Job drawing, mm, ordinate dimensions from the low corner. One solid piece. A direction names the side the tool comes from. Round coordinates to 2 decimals unless told otherwise and drop trailing zeros. Write each loop counter-clockwise with the first axis right and the second up, starting at its lowest first coordinate (ties: lowest second). Pieces come first, ordered by that corner, then holes. Notation, with made-up numbers: (24.5, 3.5) -> (41.5, 3.5) arc R19 ccw to (41.5, 27.5) -> close; hole circle Ø11 at (-16.5, -31). An arc over 180 degrees is marked (long way). Use CSV: the item, a comma, the result in double quotes. Start each with the question number.
(1) Saw through at D-D (z = 40). Give the cut face in (x, y), plus the area to 3 significant figures.
(2) Saw through at C-C (y = 14.5). Give the cut face in (x, z).
(3) Saw through at B-B (x = 51). Give the cut face in (y, z).
(4) Probe line 1 (Y direction, x = 5, z = 18); line 2 (Z direction, x = 14, y = 12.5); line 3 (Y direction, x = 63.5, z = 56.15). List the from-to ranges inside material, lowest first. Write a range as [from, to].
(5) Two-plate mould, pull along Z, no slides. Class the marked faces 5, 6 and 7: released by +Z, released by -Z, zero draft, split by the parting line, or undercut.
(6) Which spindle directions (+Z, -Z, +X, -X, +Y, -Y) get a long thin tool onto all of the face, cutting with end or side? Do the marked faces 1, 2, 3 and 4. Say none if no direction does.
(7) Saw through at A-A (x = 5). Give the cut face in (y, z), plus the area to 3 significant figures.
(8) Drop flat-ended pins along their axis: pin 1 (5.5 mm diameter, centred on x = 5, y = 14.5, fed in from +Z); pin 2 (12 mm diameter, centred on x = 23.5, z = 49, fed in from -Y); pin 3 (6 mm diameter, centred on y = 13.5, z = 44, fed in from +X); pin 4 (5.5 mm diameter, centred on y = 4.5, z = 31.5, fed in from -X). Give the stop position or say it passes through.
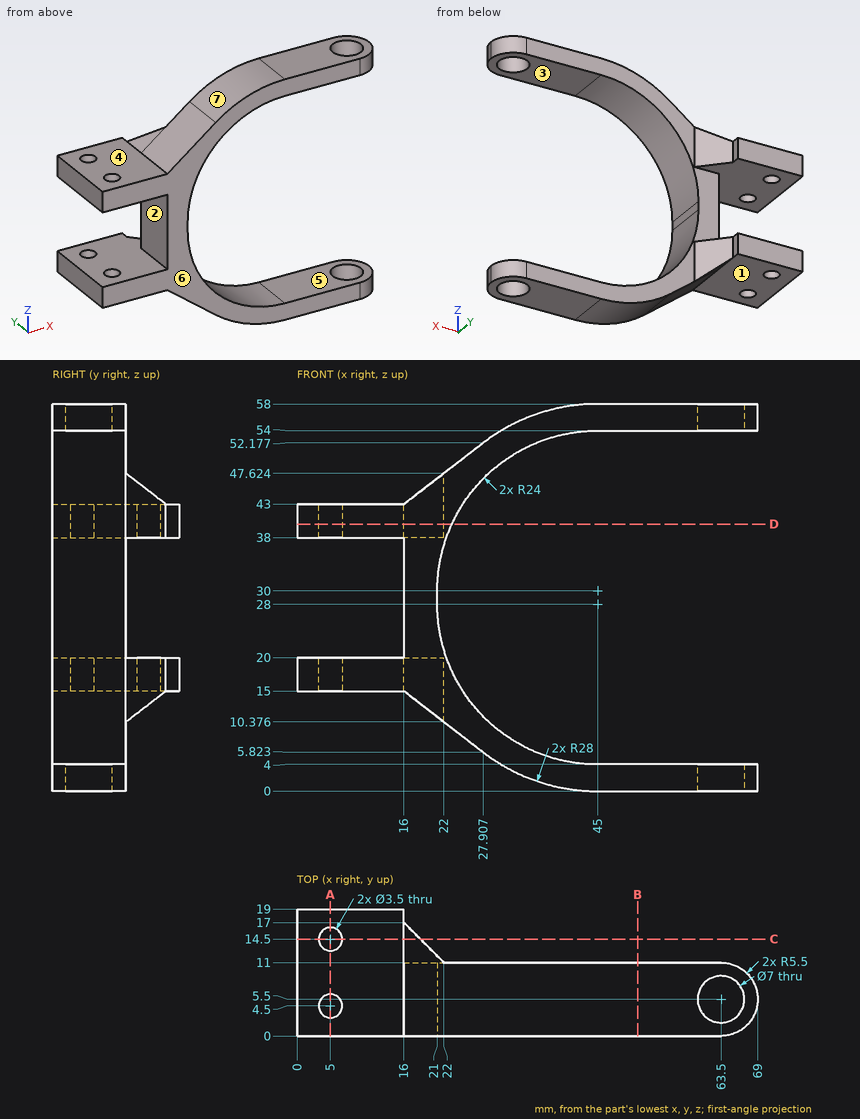
Answers:
1,outline,"(0, 0) -> (23.18, 0) -> (23.18, 11) -> (22, 11) -> (16, 17) -> (16, 19) -> (0, 19) -> close; hole circle Ø3.5 at (5, 4.5); hole circle Ø3.5 at (5, 14.5)"
1,area,"382 mm²"
2,outline,"(0, 15) -> (3.25, 15) -> (3.25, 20) -> (0, 20) -> close; (0, 38) -> (3.25, 38) -> (3.25, 43) -> (0, 43) -> close; (6.75, 15) -> (16, 15) -> (18.5, 13.07) -> (18.5, 20) -> (6.75, 20) -> close; (6.75, 38) -> (18.5, 38) -> (18.5, 44.93) -> (16, 43) -> (6.75, 43) -> close"
3,outline,"(0, 0) -> (11, 0) -> (11, 4) -> (0, 4) -> close; (0, 54) -> (11, 54) -> (11, 58) -> (0, 58) -> close"
4,line 1,"y = [0, 2.75], [6.25, 12.75], [16.25, 19]"
4,line 2,"z = [15, 20], [38, 43]"
4,line 3,"y = [0, 2], [9, 11]"
5,face 5,"undercut"
5,face 6,"zero draft"
5,face 7,"released by +Z"
6,face 1,"-Z, -X, +Y, -Y"
6,face 2,"-X, +Y, -Y"
6,face 3,"+X, +Y, -Y"
6,face 4,"+Z, -X, +Y, -Y"
7,outline,"(0, 15) -> (2.75, 15) -> (2.75, 20) -> (0, 20) -> close; (0, 38) -> (2.75, 38) -> (2.75, 43) -> (0, 43) -> close; (6.25, 15) -> (12.75, 15) -> (12.75, 20) -> (6.25, 20) -> close; (6.25, 38) -> (12.75, 38) -> (12.75, 43) -> (6.25, 43) -> close; (16.25, 15) -> (19, 15) -> (19, 20) -> (16.25, 20) -> close; (16.25, 38) -> (19, 38) -> (19, 43) -> (16.25, 43) -> close"
7,area,"120 mm²"
8,pin 1,"stops at z = 43"
8,pin 2,"stops at y = 0"
8,pin 3,"stops at x = 26.81"
8,pin 4,"stops at x = 16"
